from build123d import *

# Parameters (mm, degrees)
F0_R     = 15.875
F1_DEPTH = 19.05
F2_R     = 4.7625
F3_DEPTH = 53.975
F5_DEPTH = 6.35
F7_DEPTH = 6.35


with BuildPart() as f1:
    # F0 (on Front) → F1 (new body)
    with BuildSketch(Plane.XZ):
        with BuildLine():
            ThreePointArc((-24.250386, 93.899172), (-19.6918, 33.855441), (-41.842636, -22.138942))
            ThreePointArc((-41.842636, -22.138942), (-48.508999, -35.86211), (-50.8, -50.945779))
            Line((-50.8, -50.945779), (-38.1, -50.945779))
            ThreePointArc((-38.1, -50.945779), (0, -12.845779), (38.1, -50.945779))
            Line((38.1, -50.945779), (50.8, -50.945779))
            ThreePointArc((50.8, -50.945779), (48.508999, -35.86211), (41.842636, -22.138942))
            ThreePointArc((41.842636, -22.138942), (19.6918, 33.855441), (24.250386, 93.899172))
            ThreePointArc((24.250386, 93.899172), (0, 126.854221), (-24.250386, 93.899172))
        make_face()
        with Locations((0, 101.454221)):
            Circle(F0_R, mode=Mode.SUBTRACT)
    extrude(amount=F1_DEPTH)

    # F2 (on Top) → F3 (cut)
    with BuildSketch(Plane.XY):
        with Locations((-44.45, -9.525)):
            Circle(F2_R)
        with Locations((44.45, -9.525)):
            Circle(F2_R)
    extrude(amount=-F3_DEPTH, mode=Mode.SUBTRACT)

    # F4 (on Front) → F5 (cut)
    with BuildSketch(Plane.XZ):
        with BuildLine():
            ThreePointArc((-16.837664, 76.2), (-16.367797, 37.417239), (-26.57924, 0))
            ThreePointArc((-26.57924, 0), (-25.171809, -7.381909), (-17.79823, -8.832344))
            ThreePointArc((-17.79823, -8.832344), (0, -5.225779), (17.79823, -8.832344))
            ThreePointArc((17.79823, -8.832344), (25.171809, -7.381909), (26.57924, 0))
            ThreePointArc((26.57924, 0), (16.367797, 37.417239), (16.837664, 76.2))
            ThreePointArc((16.837664, 76.2), (14.595118, 81.720839), (8.67256, 82.378091))
            ThreePointArc((8.67256, 82.378091), (0, 80.499221), (-8.67256, 82.378091))
            ThreePointArc((-8.67256, 82.378091), (-14.595118, 81.720839), (-16.837664, 76.2))
        make_face()
    extrude(amount=F5_DEPTH, mode=Mode.SUBTRACT)

    # F6 (on face) → F7 (cut)
    with BuildSketch(Plane.XZ.offset(19.05)):
        with BuildLine():
            ThreePointArc((-16.837665, 76.200008), (-16.367858, 37.417212), (-26.579377, -4.3e-05))
            ThreePointArc((-26.579377, -4.3e-05), (-24.918717, -8.953005), (-16.011589, -10.84414))
            ThreePointArc((-16.011589, -10.84414), (-0.00013, -7.765779), (16.011348, -10.844044))
            ThreePointArc((16.011348, -10.844044), (24.918437, -8.952885), (26.579103, 4.3e-05))
            ThreePointArc((26.579103, 4.3e-05), (16.367736, 37.417266), (16.837662, 76.199992))
            ThreePointArc((16.837662, 76.199992), (14.595121, 81.720837), (8.67256, 82.378091))
            ThreePointArc((8.67256, 82.378091), (0, 80.499221), (-8.67256, 82.378091))
            ThreePointArc((-8.67256, 82.378091), (-14.595115, 81.720842), (-16.837665, 76.200008))
        make_face()
    extrude(amount=-F7_DEPTH, mode=Mode.SUBTRACT)


solid = f1.part
The listing builds one solid part. Answer for the finished solid, in the listing's coordinates (mm). A direction names the side the tool comes from. Coordinates: 2 decimals unless noted, no trailing zeros. Write each loop counter-clockwise with the first axis right and the second up, starting at its lowest first coordinate (ties: lowest second). Pieces come first, ordered by that corner, then holes. Notation, with made-up numbers: (39, -36) - (59, -36) arc R14 cw to (59, -29) - close; hole circle Ø5 at (48, -11). An arc over 180 degrees is marked (long way). Answer as CSV lines item,"result".
1. Given P1, Ø1.5, axis at y = -13, z = -21, coming from the +X side; P2, Ø4, axis at y = -12.5, z = -4, coming from the -X side; P3, Ø3, axis at x = 6, z = 61, coming from the +Y side, each flat-ended and moving along its own axis, determine where each tip first touches the part or whether it passes through.
Computed values:
P1,"stops at x = 41.54"
P2,"stops at x = -32.32"
P3,"stops at y = -6.35"
2. Find section D-D (z = 98). Give the vertices of the cut face in (x, y).
Computed values:
outline,"(-25.16, -19.05) - (-15.49, -19.05) - (-15.49, 0) - (-25.16, 0) - close; (15.49, -19.05) - (25.16, -19.05) - (25.16, 0) - (15.49, 0) - close"
3. Find section C-C (z = 11). Give the vertices of the cut face in (x, y), plus the area to 3 significant figures.
Computed values:
outline,"(-25.24, -19.05) - (-22.39, -19.05) - (-22.39, -12.7) - (22.39, -12.7) - (22.39, -19.05) - (25.24, -19.05) - (25.24, 0) - (22.39, 0) - (22.39, -6.35) - (-22.39, -6.35) - (-22.39, 0) - (-25.24, 0) - close"
area,"393 mm²"
4. A tool of negligible diameter and unlimited length cuts with its end or side. For faces 4 (the cylindrical face through (16.438, -3.131, 36.877)), 5 (the cylindrical face through (49.46, -9.39, -39.35)), 6 (the cylindrical face through (14.66, -15.92, 81.67)), from which of +Z, -Z, +X, -X, +Y, -Y can it reach the whole face along a straight path? Write none if from no direction.
Computed values:
face 4,"+Y"
face 5,"+Z, +X, +Y, -Y"
face 6,"-Y"
5. Straight lines are drawn through the part: line 1 (Y direction, x = 44.45, z = -41.5); line 2 (Z direction, x = 0, y = -8.5); line 3 (Z direction, x = -9, y = -14). For each, find the intervals that lie inside material, in ascending order. Write a range as [from, to].
Computed values:
line 1,"y = [-19.05, -14.29], [-4.76, 0]"
line 2,"z = [-12.85, 85.58], [117.33, 126.85]"
line 3,"z = [-13.92, -8.71], [82.52, 88.38], [114.53, 125.21]"
6. Find section B-B (x = 22.5). Give the vertices of the cut face in (y, z), plus the area to 3 significant figures.
Computed values:
outline,"(-19.05, -20.2) - (0, -20.2) - (0, -9.03) - (-6.35, -9.03) - (-6.35, 10.68) - (0, 10.68) - (0, 20.18) - (-19.05, 20.18) - (-19.05, 10.68) - (-12.7, 10.68) - (-12.7, -10.67) - (-19.05, -10.67) - close; (-19.05, 87.77) - (0, 87.77) - (0, 113.24) - (-19.05, 113.24) - close"
area,"994 mm²"
7. Determine the mould class of faces 1 (the cylindrical face through (-16.3, -3.13, 37.96)), 2 (the flat face through (0, -12.7, 26)), 3 (the cylindrical face through (39.69, -9.32, -38.26)) for opening direction Y: +Y half, -Y half, draft (parallel to the pull), parting line (faces both ways), or undercut.
Computed values:
face 1,"draft"
face 2,"-Y half"
face 3,"undercut"
